Input: dimensioned drawing with shaded views. Units: mm. Origin: part minimum x, y, z. A direction names the side the tool comes from. Round coordinates to 2 decimals unless told otherwise and drop trailing zeros. Loops run counter-clockwise (first coordinate to the right, second up) from the corner with the lowest first, then second, coordinate; pieces in that order, holes last.
1) Section A-A, the plane y = 3.5. Return loops of the section in (x, z), and give its area (3 significant figures).
2) First-contact query: pin 1 (1.6 mm diameter, centred on x = 12.55, z = 7.05, fed in from -Y). Flat tip, straight axial feed; report the tip coordinate or a pass-through.
3) Ray query, line 1 along Z through (x, y) = (3.55, 1.8); line 2 along X through (y, z) = (2.25, 3.5); line 3 along Z through (x, y) = (7, 5.5). Return the intervals inside material, ascending.
4) Draft query along Z for the marked faces 1, 2, 3 and 4. Return one class per face: pulls with the +Z half, pulls with the -Z half, needs draft (parallel to the pull), parting line crosses it, or undercut.
5) Access query for the marked faces 5 and 6. Directions: +Z, -Z, +X, -X, +Y, -Y. A direction counts if a zero-diameter tool reaches every point of the face in a straight line with its end or side. Return the directions, or none.
6) Section B-B, the plane x = 3.55. Return loops of the section in (y, z), and give its area (3 significant figures).
7) Section C-C, the plane z = 7.05. Return loops of the section in (x, y).
8) Section D-D, the plane z = 4. Return loops of the section in (x, y).
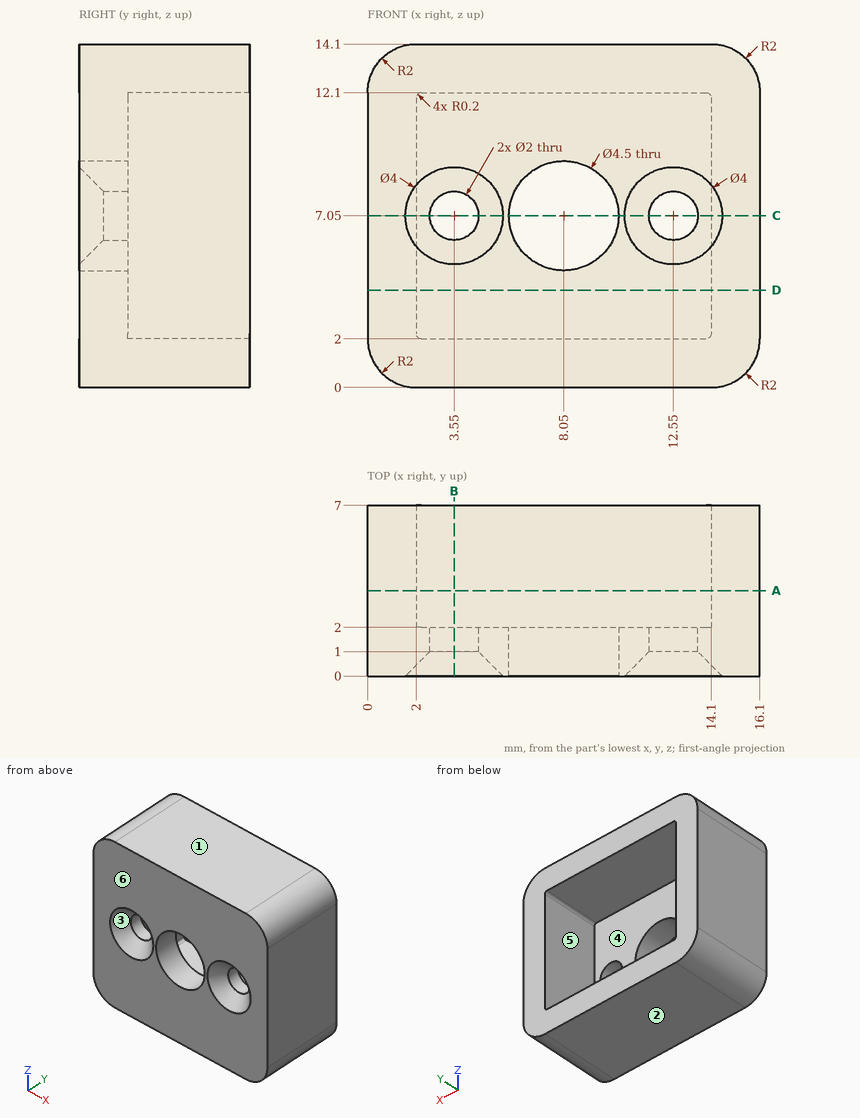
Final values:
1. outline: (0, 2) arc R2 ccw to (2, 0) - (14.1, 0) arc R2 ccw to (16.1, 2) - (16.1, 12.1) arc R2 ccw to (14.1, 14.1) - (2, 14.1) arc R2 ccw to (0, 12.1) - close; hole (2, 2.2) arc R0.2 ccw to (2.2, 2) - (13.9, 2) arc R0.2 ccw to (14.1, 2.2) - (14.1, 11.9) arc R0.2 ccw to (13.9, 12.1) - (2.2, 12.1) arc R0.2 ccw to (2, 11.9) - close
1. area: 101 mm2
2. pin 1: passes through
3. line 1: z = 0 to 6.05, 8.05 to 14.1
3. line 2: x = 0 to 2, 14.1 to 16.1
3. line 3: z = 0 to 2, 12.1 to 14.1
4. face 1: pulls with the +Z half
4. face 2: pulls with the -Z half
4. face 3: undercut
4. face 4: undercut
5. face 5: +Y
5. face 6: +Z, -Z, +X, -X, -Y
6. outline: (0, 0) - (7, 0) - (7, 2) - (2, 2) - (2, 6.05) - (1, 6.05) - (0, 5.05) - close; (0, 9.05) - (1, 8.05) - (2, 8.05) - (2, 12.1) - (7, 12.1) - (7, 14.1) - (0, 14.1) - close
6. area: 43.2 mm2
7. outline: (0, 0) - (1.55, 0) - (2.55, 1) - (2.55, 2) - (2, 2) - (2, 7) - (0, 7) - close; (4.55, 1) - (5.55, 0) - (5.8, 0) - (5.8, 2) - (4.55, 2) - close; (10.3, 0) - (10.55, 0) - (11.55, 1) - (11.55, 2) - (10.3, 2) - close; (13.55, 1) - (14.55, 0) - (16.1, 0) - (16.1, 7) - (14.1, 7) - (14.1, 2) - (13.55, 2) - close
8. outline: (0, 0) - (16.1, 0) - (16.1, 7) - (14.1, 7) - (14.1, 2) - (2, 2) - (2, 7) - (0, 7) - close
